Source: CAD feature listing. Evaluate the final solid. Frame: model axes, mm. Face numbers are marked on the shaded views. Round coordinates to 2 decimals unless told otherwise and drop trailing zeros. Loops run counter-clockwise (first coordinate to the right, second up) from the corner with the lowest first, then second, coordinate; pieces in that order, holes last. Notation, with made-up numbers: (63, -35) - (115, -35) arc R25 cw to (115, -5) - close; hole circle Ø11 at (11.25, 27.5). An arc over 180 degrees is marked (long way). Write item = value, one per line. Start each with the question number.
from build123d import *

# Parameters (mm, degrees)
SKETCH_1_W      = 600
SKETCH_1_H      = 600
EXTRUDE_1_DEPTH = 30
SKETCH_2_W      = 50
SKETCH_2_H      = 50
EXTRUDE_2_DEPTH = 800


with BuildPart() as part:
    # 草图1 → 凸台-拉伸1 (new body)
    with BuildSketch(Plane(origin=(0, 0, 0), x_dir=(1, 0, 0), z_dir=(0, 1, 0))):
        Rectangle(SKETCH_1_W, SKETCH_1_H)
    extrude(amount=EXTRUDE_1_DEPTH)

    # 草图2 → 凸台-拉伸2 (add)
    with BuildSketch(Plane.XZ):
        with Locations((-275, 275)):
            Rectangle(SKETCH_2_W, SKETCH_2_H)
        with Locations((275, 275)):
            Rectangle(SKETCH_2_W, SKETCH_2_H)
        with Locations((275, -275)):
            Rectangle(SKETCH_2_W, SKETCH_2_H)
        with Locations((-275, -275)):
            Rectangle(SKETCH_2_W, SKETCH_2_H)
    extrude(amount=EXTRUDE_2_DEPTH)


solid = part.part
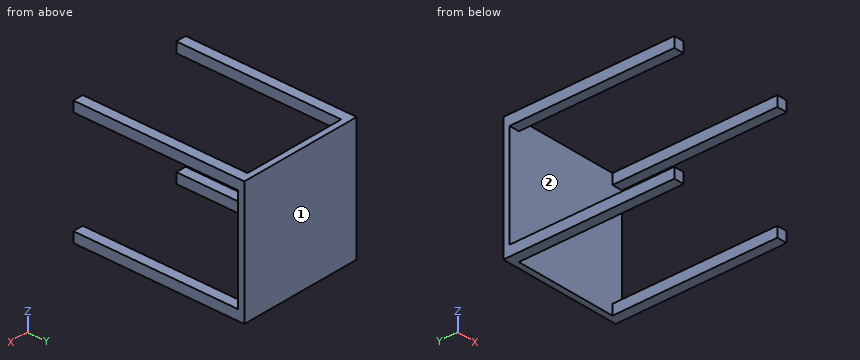
(1) Mould query, pull axis X, two halves, no side actions, for the marked faces 1 and 2. Classes: +X half, -X half, draft (parallel to the pull), parting line (faces both ways), or undercut.
(2) Material intervals for line 1 along X through (y, z) = (-152, -260); line 2 along Y through (x, z) = (92.5, 2), sorted ascending. Write a range as from..to.
(3) Cut plane A-A (y = -59.5). Output: boundary loops of the cut face in (x, z), and give its area (3 significant figures).
(4) Cut plane C-C (x = -175.5). Output: boundary loops of the cut face in (y, z).
(5) Cut plane B-B (z = -155.5). Output: boundary loops of the cut face in (x, y), and give its area (3 significant figures).
Solution:
q1.face_1 = draft
q1.face_2 = undercut
q2.line_1 = -300..-250, 250..300
q2.line_2 = 0..30
q3.outline = (-300, -300) - (-250, -300) - (-250, -250) - (-300, -250) - close; (-300, 250) - (-250, 250) - (-250, 300) - (-300, 300) - close; (250, -300) - (300, -300) - (300, -250) - (250, -250) - close; (250, 250) - (300, 250) - (300, 300) - (250, 300) - close
q3.area = 10,000 mm^2
q4.outline = (0, -300) - (30, -300) - (30, 300) - (0, 300) - close
q5.outline = (-300, 0) - (300, 0) - (300, 30) - (-300, 30) - close
q5.area = 18,000 mm^2
